from build123d import *

# Parameters (mm, degrees)
F3_W      = 890.734077
F3_H      = 1319.233716
F4_DEPTH  = 254
F6_W      = 1012.359947
F6_H      = 1290.58224
F7_DEPTH  = 254
F10_DEPTH = 254
F12_W     = 1270.54733
F12_H     = 1196.680188
F13_DEPTH = 254
F15_W     = 950.985431
F15_H     = 1887.960911
F16_DEPTH = 254
F19_DEPTH = 254
F20_R     = 101.6
F21_DEPTH = 152.4


with BuildPart() as f1:
    # F0 (on Front) → F1 (revolve)
    with BuildSketch(Plane.XZ):
        with BuildLine():
            Line((-359.156, 0), (0, 0))
            Line((0, 0), (359.156, 0))
            ThreePointArc((359.156, 0), (0, 359.156), (-359.156, 0))
        make_face()
    revolve(axis=Axis((179.578, 0, 0), (1, 0, 0)))

    # F3 (on offset) → F4 (cut)
    with BuildSketch(Plane.XZ.offset(254)):
        with Locations((-42.36114, 63.51766)):
            Rectangle(F3_W, F3_H)
    extrude(amount=F4_DEPTH, mode=Mode.SUBTRACT)

    # F6 (on offset) → F7 (cut)
    with BuildSketch(Plane.XZ.offset(-254)):
        with Locations((-90.278938, 130.936891)):
            Rectangle(F6_W, F6_H)
    extrude(amount=-F7_DEPTH, mode=Mode.SUBTRACT)

    # F9 (on offset) → F10 (cut)
    with BuildSketch(Plane.XY.offset(254)):
        Polygon((-582.261324, -515.396833), (446.441472, -515.396833), (446.441472, -508.58891), (456.421018, -508.58891), (456.421018, 446.415097), (-582.261324, 446.415097), align=None)
    extrude(amount=F10_DEPTH, mode=Mode.SUBTRACT)

    # F12 (on offset) → F13 (cut)
    with BuildSketch(Plane.XY.offset(-254)):
        with Locations((82.284361, 80.805302)):
            Rectangle(F12_W, F12_H)
    extrude(amount=-F13_DEPTH, mode=Mode.SUBTRACT)

    # F15 (on offset) → F16 (cut)
    with BuildSketch(Plane.YZ.offset(-254)):
        with Locations((-55.342019, -317.589998)):
            Rectangle(F15_W, F15_H)
    extrude(amount=-F16_DEPTH, mode=Mode.SUBTRACT)

    # F18 (on offset) → F19 (cut)
    with BuildSketch(Plane.YZ.offset(254)):
        Polygon((-462.633133, 1110.26144), (-462.633133, 1077.45111), (-462.633133, -1249.087334), (636.57546, -1249.087334), (636.57546, 1110.26144), align=None)
    extrude(amount=F19_DEPTH, mode=Mode.SUBTRACT)

    # F20 (on face) → F21 (cut)
    with BuildSketch(Plane.XY.offset(254)):
        Circle(F20_R)
    extrude(amount=-F21_DEPTH, mode=Mode.SUBTRACT)


solid = f1.part
Can you work these out from the model? Positions are in its coordinate system, mm. Coordinates: 2 decimals unless noted, no trailing zeros. Loops run counter-clockwise (first coordinate to the right, second up) from the corner with the lowest first, then second, coordinate; pieces in that order, holes last. Notation, with made-up numbers: M -2,33 L 53,33 A20 ccw 53,61 Z; hole C 10,5 d6. An arc over 180 degrees is marked long. Return JSON: item names as keys, results as strings. Group by question number.
Item 1: Imagine slicing it at D-D (x = 185). Please give me the cut outline in (y, z).
Item 2: Thinking about a two-plate mould opening in X: for faces 1 (the flat face through (-254, -4, 4)), 2 (the flat face through (-1, 1, 101.6)), 3 (the cylindrical face through (-22.025, -99.184, 178.867)), 4 (the flat face through (109, 4, 254)), which applies, released by +X, released by -X, zero draft, split by the parting line, or undercut?
Item 3: If I drill on L1, parallel to Y at x = 0, z = 185; L2, parallel to Y at x = 37, z = 151; L3, parallel to X at y = -52, z = 136, over which ranges is the centre line in solid material (lowest first)? Write a range as from..to.
Item 4: Imagine slicing it at C-C (z = -171). Please give me the cut outline in (x, y).
Item 5: Imagine slicing it at A-A (x = 0). Please give me the cut outline in (y, z), and give its area (3 significant figures).
Verdict:
{
 "1": {"outline": "M -254,-173.93 A307.84 ccw -173.93,-254 L 173.93,-254 A307.84 ccw 254,-173.93 L 254,173.93 A307.84 ccw 173.93,254 L -173.93,254 A307.84 ccw -254,173.93 Z"},
 "2": {"face 1": "released by -X", "face 2": "undercut", "face 3": "undercut", "face 4": "zero draft"},
 "3": {"L1": "y = -254..-101.6, 101.6..254", "L2": "y = -254..-94.62, 94.62..254", "L3": "x = -254..-87.28, 87.28..254"},
 "4": {"outline": "M -254,-187.71 A315.84 ccw -187.71,-254 L 187.71,-254 A315.84 ccw 254,-187.71 L 254,187.71 A315.84 ccw 187.71,254 L -187.71,254 A315.84 ccw -254,187.71 Z"},
 "5": {"outline": "M -254,-253.92 A359.16 ccw -253.92,-254 L 253.92,-254 A359.16 ccw 254,-253.92 L 254,253.92 A359.16 ccw 253.92,254 L 101.6,254 L 101.6,101.6 L -101.6,101.6 L -101.6,254 L -253.92,254 A359.16 ccw -254,253.92 Z", "area": "227,000 mm^2"}
}
